Read the model definition and answer for the solid it produces. Units are mm, in the model's axes. Round coordinates to 2 decimals unless told otherwise and drop trailing zeros. Write each loop counter-clockwise with the first axis right and the second up, starting at its lowest first coordinate (ties: lowest second). Pieces come first, ordered by that corner, then holes. Notation, with made-up numbers: (31, 78) -> (85, 78) arc R22 ccw to (85, 104) -> close; hole circle Ø6 at (81.25, 47). An arc over 180 degrees is marked (long way). Return JSON: item names as keys, results as strings. Group by question number.
(1) A cutting plane is placed at A-A on z = 1. Give the vertices of the cut face in (x, y).
(2) Given pin 1 (6 mm diameter, centred on x = -11.5, y = -24.5, fed in from -Z), flat-ended and moving along its own axis, determine where the tip first touches the part or whether it passes through.
(3) Straight lines are drawn through the part: line 1 (Y direction, x = -17, z = 7.75); line 2 (X direction, y = -24, z = 9); line 3 (X direction, y = -37.5, z = 0.75). For each, find the intervals that lie inside material, in ascending order.
(4) A cutting plane is placed at B-B on x = -36. Give the vertices of the cut face in (y, z), then the cut area to 3 significant figures.
(5) A cutting plane is placed at C-C on y = 2. Give the vertices of the cut face in (x, z).
```python
from build123d import *

# Parameters (mm, degrees)
F0_W     = 90
F0_H     = 84
F1_DEPTH = 10
F2_W     = 83
F2_H     = 76.2
F2_W_2   = 76.2
F2_H_2   = 69.5
F3_DEPTH = 3.2
F4_W     = 83
F4_H     = 76.2
F4_W_2   = 76.2
F4_H_2   = 69.5
F5_DEPTH = 3.2


with BuildPart() as f1:
    # F0 (on Top) → F1 (new body)
    with BuildSketch(Plane.XY):
        Rectangle(F0_W, F0_H)
    extrude(amount=F1_DEPTH)

    # F2 (on face) → F3 (cut)
    with BuildSketch(Plane.XY.offset(10)):
        Rectangle(F2_W, F2_H)
        Rectangle(F2_W_2, F2_H_2, mode=Mode.SUBTRACT)
    extrude(amount=-F3_DEPTH, mode=Mode.SUBTRACT)

    # F4 (on face) → F5 (cut)
    with BuildSketch(Plane(origin=(0, 0, 0), x_dir=(1, 0, 0), z_dir=(0, 0, -1))):
        Rectangle(F4_W, F4_H)
        Rectangle(F4_W_2, F4_H_2, mode=Mode.SUBTRACT)
    extrude(amount=-F5_DEPTH, mode=Mode.SUBTRACT)


solid = f1.part
```
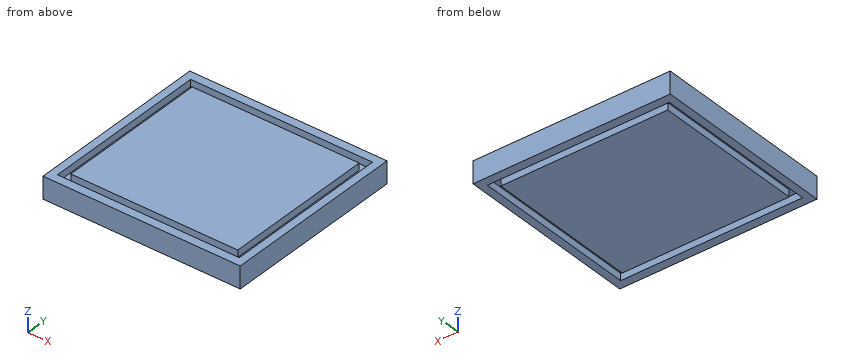
Checks:
{
 "1": {"outline": "(-45, -42) -> (45, -42) -> (45, 42) -> (-45, 42) -> close; (-38.1, -34.75) -> (38.1, -34.75) -> (38.1, 34.75) -> (-38.1, 34.75) -> close; hole (-41.5, -38.1) -> (41.5, -38.1) -> (41.5, 38.1) -> (-41.5, 38.1) -> close"},
 "2": {"pin 1": "stops at z = 0"},
 "3": {"line 1": "y = -42 to -38.1, -34.75 to 34.75, 38.1 to 42", "line 2": "x = -45 to -41.5, -38.1 to 38.1, 41.5 to 45", "line 3": "x = -45 to -41.5, 41.5 to 45"},
 "4": {"outline": "(-42, 0) -> (-38.1, 0) -> (-38.1, 3.2) -> (-34.75, 3.2) -> (-34.75, 0) -> (34.75, 0) -> (34.75, 3.2) -> (38.1, 3.2) -> (38.1, 0) -> (42, 0) -> (42, 10) -> (38.1, 10) -> (38.1, 6.8) -> (34.75, 6.8) -> (34.75, 10) -> (-34.75, 10) -> (-34.75, 6.8) -> (-38.1, 6.8) -> (-38.1, 10) -> (-42, 10) -> close", "area": "797 mm^2"},
 "5": {"outline": "(-45, 0) -> (-41.5, 0) -> (-41.5, 3.2) -> (-38.1, 3.2) -> (-38.1, 0) -> (38.1, 0) -> (38.1, 3.2) -> (41.5, 3.2) -> (41.5, 0) -> (45, 0) -> (45, 10) -> (41.5, 10) -> (41.5, 6.8) -> (38.1, 6.8) -> (38.1, 10) -> (-38.1, 10) -> (-38.1, 6.8) -> (-41.5, 6.8) -> (-41.5, 10) -> (-45, 10) -> close"}
}
